The listing builds one solid part. Answer for the finished solid, in the listing's coordinates (mm). A direction names the side the tool comes from. Give positions to 0.01 mm unless a question says otherwise; leave off trailing zeros. Write each loop counter-clockwise with the first axis right and the second up, starting at its lowest first coordinate (ties: lowest second). Pieces come first, ordered by that corner, then holes. Notation, with made-up numbers: (48.5, -26.5) -> (104.5, -26.5) arc R17 cw to (104.5, -17.5) -> close; hole circle Ø9 at (33, 78.5). An arc over 180 degrees is marked (long way). Put each result on its own line as item: value. Start each with the question number.
1) For a pull along Y with two mould halves and no side action, classify faces 1 (the flat face through (127, -51, -17)), 2 (the flat face through (62.611, -20.845, -28.735)), 3 (the flat face through (62.611, -29.465, 19.799)) as released by +Y, released by -Y, zero draft, split by the parting line, or undercut.
2) A cutting plane is placed at C-C (z = -52.5). Write down the section's boundary in (x, y), then the cut area to 3 significant figures.
3) For faces 4 (the flat face through (62.611, -44.047, 36.833)), 5 (the flat face through (0, -51, -17)), 6 (the flat face through (63, -33.933, -73)), 7 (the flat face through (63, -67.393, -17)), 8 (the flat face through (62.61, -26.68, 5.72)), determine the directions among +Z, -Z, +X, -X, +Y, -Y from which every point of the face is accessible in a straight line to the end or side of a thin tool.
4) A cutting plane is placed at D-D (z = -32.5). Write down the section's boundary in (x, y), then the cut area to 3 significant figures.
5) A cutting plane is placed at B-B (z = 21). Write down the section's boundary in (x, y), then the cut area to 3 significant figures.
6) Flat-ended cylindrical pins translate along their axes: pin 1 Ø15 at (x, z) = (48, -65) entering from +Y; pin 2 Ø8 at (x, z) = (44.5, 45) entering from +Y; pin 3 Ø10 at (x, z) = (29, -38.5) entering from +Y; pin 4 Ø10 at (x, y) = (87.5, -32) entering from -Z. Find the tip coordinate at first contact, or state that the pin passes through.
7) Find the intervals of material crossed by line 1 along Y through (x, z) = (8.5, 32.5); line 2 along Y through (x, z) = (41, 8.5); line 3 along Z through (x, y) = (91, -14.5), in increasing order. Write a range as from..to.
8) A cutting plane is placed at A-A (x = 97). Write down the section's boundary in (y, z), then the cut area to 3 significant figures.
from build123d import *

# Parameters (mm, degrees)
F1_DEPTH = 127


with BuildPart() as f1:
    # F0 (on Right) → F1 (new body)
    with BuildSketch(Plane.YZ):
        with BuildLine():
            Line((-48.929181, 61.623078), (-67.393027, 61.623078))
            Line((-67.393027, 61.623078), (-67.393027, -98.089159))
            Line((-67.393027, -98.089159), (-33.93315, -98.089159))
            Line((-33.93315, -98.089159), (-33.93315, -47.811495))
            Line((-33.93315, -47.811495), (-7.385537, -9.11652))
            ThreePointArc((-7.385537, -9.11652), (-7.800447, -1.53815), (-15.232671, 0))
            Line((-15.232671, 0), (-26.310977, -18.23304))
            ThreePointArc((-26.310977, -18.23304), (-33.618065, -21.605825), (-36.466088, -14.078676))
            Line((-36.466088, -14.078676), (-16.617458, 26.080182))
            ThreePointArc((-16.617458, 26.080182), (-15.863933, 34.392833), (-24.002995, 32.542527))
            Line((-24.002995, 32.542527), (-35.081301, 6.693146))
            ThreePointArc((-35.081301, 6.693146), (-41.501132, 5.135256), (-43.851625, 11.309107))
            Line((-43.851625, 11.309107), (-32.77332, 40.851254))
            ThreePointArc((-32.77332, 40.851254), (-33.374387, 49.612313), (-41.543644, 46.390408))
            Line((-41.543644, 46.390408), (-46.621203, 27.003372))
            ThreePointArc((-46.621203, 27.003372), (-52.936608, 25.304014), (-55.853125, 31.157738))
            Line((-55.853125, 31.157738), (-48.929181, 61.623078))
        make_face()
    extrude(amount=F1_DEPTH)


solid = f1.part
Reply:
1. face 1: zero draft
1. face 2: released by +Y
1. face 3: undercut
2. outline: (0, -67.39) -> (127, -67.39) -> (127, -33.93) -> (0, -33.93) -> close
2. area: 4,250 mm2
3. face 4: +Z, +X, -X
3. face 5: +Z, -Z, -X, +Y, -Y
3. face 6: -Z, +X, -X, +Y
3. face 7: +Z, -Z, +X, -X, -Y
3. face 8: +X, -X
4. outline: (0, -67.39) -> (127, -67.39) -> (127, -23.43) -> (0, -23.43) -> close
4. area: 5,580 mm2
5. outline: (0, -67.39) -> (127, -67.39) -> (127, -40.22) -> (0, -40.22) -> close; (0, -28.95) -> (127, -28.95) -> (127, -19.13) -> (0, -19.13) -> close
5. area: 4,700 mm2
6. pin 1: stops at y = -33.93
6. pin 2: stops at y = -30.84
6. pin 3: stops at y = -24.11
6. pin 4: stops at z = -98.09
7. line 1: y = -67.39..-55.55, -45.18..-35.91, -24.02..-14.5
7. line 2: y = -67.39..-44.06, -34.31..-25.31
7. line 3: z = -19.49..0.3, 28.52..32.5
8. outline: (-67.39, -98.09) -> (-33.93, -98.09) -> (-33.93, -47.81) -> (-7.39, -9.12) arc R6.22 ccw to (-15.23, 0) -> (-26.31, -18.23) arc R5.5 cw (long way) to (-36.47, -14.08) -> (-16.62, 26.08) arc R5.16 ccw (long way) to (-24, 32.54) -> (-35.08, 6.69) arc R4.99 cw to (-43.85, 11.31) -> (-32.77, 40.85) arc R5.44 ccw (long way) to (-41.54, 46.39) -> (-46.62, 27) arc R5.16 cw to (-55.85, 31.16) -> (-48.93, 61.62) -> (-67.39, 61.62) -> close
8. area: 5,540 mm2
